from build123d import *

# Parameters (mm, degrees)
F0_W     = 235.203512
F0_H     = 118.836838
F0_R     = 9.843794
F0_W_2   = 109.183416
F0_H_2   = 48.583305
F1_DEPTH = 50.8
F2_R     = 5.08
F3_R     = 5.08
F4_R     = 5.08


with BuildPart() as f1:
    # F0 (on Front) → F1 (new body)
    with BuildSketch(Plane.XZ):
        with Locations((-7.397939, -7.492734)):
            Rectangle(F0_W, F0_H)
        with Locations((-109.693609, -52.839234)):
            Circle(F0_R, mode=Mode.SUBTRACT)
        with Locations((-17.346896, -9.089239)):
            Rectangle(F0_W_2, F0_H_2, mode=Mode.SUBTRACT)
        with Locations((91.326304, -49.401499)):
            Circle(F0_R, mode=Mode.SUBTRACT)
        with Locations((-108.162999, 34.3371)):
            Circle(F0_R, mode=Mode.SUBTRACT)
        with Locations((92.856914, 35.22383)):
            Circle(F0_R, mode=Mode.SUBTRACT)
    extrude(amount=F1_DEPTH)

    # F2
    f2_edges = [f1.edges().sort_by_distance(p)[0] for p in [
        (110.203817, -25.4, -66.911153),
        (-124.999695, -25.4, -66.911153),
    ]]
    fillet(f2_edges, radius=F2_R)

    # F3
    f3_edges = [f1.edges().sort_by_distance(p)[0] for p in [
        (-124.999695, -25.4, 51.925685),
    ]]
    fillet(f3_edges, radius=F3_R)

    # F4
    f4_edges = [f1.edges().sort_by_distance(p)[0] for p in [
        (110.203817, -25.4, 51.925685),
    ]]
    fillet(f4_edges, radius=F4_R)


solid = f1.part
Geometry: final body of the model. Coordinates: model frame, mm. A direction names the side the tool comes from. Give positions to 0.01 mm unless a question says otherwise; leave off trailing zeros. Order: outer loops, then holes, each group sorted by start corner. A loop starts at its lowest first (then second) coordinate and runs counter-clockwise, first axis right, second up. Notation, with made-up numbers: (61.5, 56.5) -> (111.5, 56.5) arc R24 cw to (111.5, 92.5) -> close; hole circle Ø1 at (18, 20). An arc over 180 degrees is marked (long way). Answer as a JSON object with one key per item and string values.
Q1. Section C-C (z = 28). Output: boundary loops of the cut face in (x, y), plus the area to 3 significant figures.
Entries:
{"outline": "(-125, -50.8) -> (-115.7, -50.8) -> (-115.7, 0) -> (-125, 0) -> close; (-100.63, -50.8) -> (86.17, -50.8) -> (86.17, 0) -> (-100.63, 0) -> close; (99.54, -50.8) -> (110.2, -50.8) -> (110.2, 0) -> (99.54, 0) -> close", "area": "10,500 mm^2"}
Q2. Section D-D (y = -4). Output: boundary loops of the cut face in (x, z).
Entries:
{"outline": "(-125, -61.83) arc R5.08 ccw to (-119.92, -66.91) -> (105.12, -66.91) arc R5.08 ccw to (110.2, -61.83) -> (110.2, 46.85) arc R5.08 ccw to (105.12, 51.93) -> (-119.92, 51.93) arc R5.08 ccw to (-125, 46.85) -> close; hole circle Ø19.69 at (-109.69, -52.84); hole circle Ø19.69 at (-108.16, 34.34); hole (-71.94, -33.38) -> (37.24, -33.38) -> (37.24, 15.2) -> (-71.94, 15.2) -> close; hole circle Ø19.69 at (91.33, -49.4); hole circle Ø19.69 at (92.86, 35.22)"}
Q3. Material intervals for probe 1 along Z at (x, y) = (92, -33); probe 2 along X at (y, z) = (-38, -9); probe 3 along Z at (x, y) = (-63.5, -48), sorted ascending.
Entries:
{"probe 1": "z = -66.91 to -59.22, -39.58 to 25.42, 45.03 to 51.93", "probe 2": "x = -125 to -71.94, 37.24 to 110.2", "probe 3": "z = -66.91 to -33.38, 15.2 to 51.93"}
Q4. Draft query along X for faces 1 (the flat face through (-9, -50.8, 20)), 2 (the flat face through (110.204, -25, -8)), 3 (the cylindrical face through (83.023, -25.044, 35.657)). Return one class per face: released by +X, released by -X, zero draft, split by the parting line, or undercut.
Entries:
{"face 1": "zero draft", "face 2": "released by +X", "face 3": "undercut"}
Q5. Section B-B (z = 7.5). Output: boundary loops of the cut face in (x, y), plus the area to 3 significant figures.
Entries:
{"outline": "(-125, -50.8) -> (-71.94, -50.8) -> (-71.94, 0) -> (-125, 0) -> close; (37.24, -50.8) -> (110.2, -50.8) -> (110.2, 0) -> (37.24, 0) -> close", "area": "6,400 mm^2"}
Q6. Access query for faces 4 (the flat face through (-18, -25, 15.202)), 5 (the cylindrical face through (108.68, -25.76, -65.46)). Directions: +Z, -Z, +X, -X, +Y, -Y. A direction counts if a zero-diameter tool reaches every point of the face in a straight line with its end or side. Return the directions, or none.
Entries:
{"face 4": "+Y, -Y", "face 5": "-Z, +X, +Y, -Y"}
Q7. Section A-A (x = 33.5). Output: boundary loops of the cut face in (y, z).
Entries:
{"outline": "(-50.8, -66.91) -> (0, -66.91) -> (0, -33.38) -> (-50.8, -33.38) -> close; (-50.8, 15.2) -> (0, 15.2) -> (0, 51.93) -> (-50.8, 51.93) -> close"}
